Verification items for the finished model (mm, model axes). Face numbers are marked on the shaded views. A direction names the side the tool comes from. Coordinates: 2 decimals unless noted, no trailing zeros. Loops run counter-clockwise (first coordinate to the right, second up) from the corner with the lowest first, then second, coordinate; pieces in that order, holes last. Notation, with made-up numbers: (-36, 15.5) - (-15, 15.5) arc R24 cw to (-15, 43.5) - close; hole circle Ø6 at (5, 29). An arc over 180 degrees is marked (long way). Answer as CSV lines item,"result". Start each with the question number.
1. Cross-section at C-C (y = 4.75). Enter the section's corners in (x, z).
2. Gauge pin test, flat end, axial feed: P1, Ø9, axis at x = 4, y = 5.5, coming from the +Z side. Record the tip position at first contact, or that the pin passes through.
3. Cross-section at B-B (z = 7.5). Enter the section's corners in (x, y).
4. Cross-section at A-A (y = -2.5). Enter the section's corners in (x, z), plus the area to 3 significant figures.
5. Material ranges on line 1 (X direction, y = 0.75, z = 4.5); line 2 (Z direction, x = -3.5, y = 6.75); line 3 (Y direction, x = 16.85, z = 7), recorded low to high. Write a range as [from, to].
6. Release check for a two-part mould opening along X. For the marked faces 1, 2 and 3 record: pulls with the +X half, pulls with the -X half, needs draft (parallel to the pull), parting line crosses it, or undercut.
7. Cross-section at D-D (x = 10.5). Enter the section's corners in (y, z), plus the area to 4 significant figures.
8. Set-up check for the marked faces 4 and 5: record each of +Z, -Z, +X, -X, +Y, -Y from which the full face is reachable in a straight line by a thin tool's end or side.
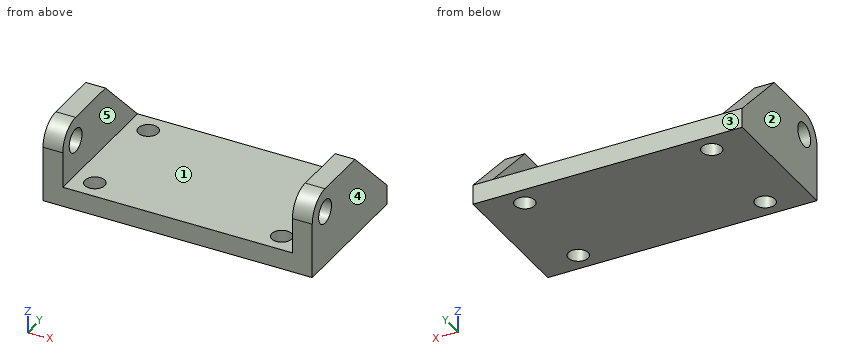
```python
from build123d import *

# Parameters (mm, degrees)
SKETCH1_W           = 34
SKETCH1_H           = 17.5
SKETCH1_R           = 1.25
BOSS_EXTRUDE1_DEPTH = 2.5
SKETCH2_W           = 2.5
SKETCH2_H           = 17.5
BOSS_EXTRUDE2_DEPTH = 7.5
CHAMFER1_SIZE       = 7.5
FILLET1_R           = 3
SKETCH3_R           = 1.5
CUT_EXTRUDE1_DEPTH  = 35


with BuildPart() as part:
    # Sketch1 → Boss-Extrude1 (new body)
    with BuildSketch(Plane.XY):
        with Locations((0.621428571, 4.137142857)):
            Rectangle(SKETCH1_W, SKETCH1_H)
        with Locations((-11.178571429, -2.112857143)):
            Circle(SKETCH1_R, mode=Mode.SUBTRACT)
        with Locations((12.421428571, -2.112857143)):
            Circle(SKETCH1_R, mode=Mode.SUBTRACT)
        with Locations((12.421428571, 10.387142857)):
            Circle(SKETCH1_R, mode=Mode.SUBTRACT)
        with Locations((-11.178571429, 10.387142857)):
            Circle(SKETCH1_R, mode=Mode.SUBTRACT)
    extrude(amount=BOSS_EXTRUDE1_DEPTH)

    # Sketch2 → Boss-Extrude2 (add)
    with BuildSketch(Plane.XY.offset(2.5)):
        with Locations((-15.128571429, 4.137142857)):
            Rectangle(SKETCH2_W, SKETCH2_H)
        with Locations((16.371428571, 4.137142857)):
            Rectangle(SKETCH2_W, SKETCH2_H)
    extrude(amount=BOSS_EXTRUDE2_DEPTH)

    # Chamfer1
    chamfer1_edges = [part.edges().sort_by_distance(p)[0] for p in [
        (16.371428571, 12.887142857, 10),
        (-15.128571429, 12.887142857, 10),
    ]]
    chamfer(chamfer1_edges, length=CHAMFER1_SIZE)

    # Fillet1
    fillet1_edges = [part.edges().sort_by_distance(p)[0] for p in [
        (-15.128571429, -4.612857143, 10),
        (16.371428571, -4.612857143, 10),
    ]]
    fillet(fillet1_edges, radius=FILLET1_R)

    # Sketch3 → Cut-Extrude1 (cut, through all)
    with BuildSketch(Plane(origin=(17.621428571, 0, 0), x_dir=(0, 0, -1), z_dir=(1, 0, 0))):
        with Locations((-7, -1.612857143)):
            Circle(SKETCH3_R)
    extrude(amount=-CUT_EXTRUDE1_DEPTH, mode=Mode.SUBTRACT)


solid = part.part
```
Values follow:
1,outline,"(-16.38, 0) - (17.62, 0) - (17.62, 10) - (15.12, 10) - (15.12, 2.5) - (-13.88, 2.5) - (-13.88, 10) - (-16.38, 10) - close"
2,P1,"stops at z = 2.5"
3,outline,"(-16.38, -4.57) - (-13.88, -4.57) - (-13.88, -3.03) - (-16.38, -3.03) - close; (-16.38, -0.2) - (-13.88, -0.2) - (-13.88, 7.89) - (-16.38, 7.89) - close; (15.12, -4.57) - (17.62, -4.57) - (17.62, -3.03) - (15.12, -3.03) - close; (15.12, -0.2) - (17.62, -0.2) - (17.62, 7.89) - (15.12, 7.89) - close"
4,outline,"(-16.38, 0) - (-12.37, 0) - (-12.37, 2.5) - (-13.88, 2.5) - (-13.88, 5.79) - (-16.38, 5.79) - close; (-16.38, 8.21) - (-13.88, 8.21) - (-13.88, 9.87) - (-16.38, 9.87) - close; (-9.99, 0) - (11.23, 0) - (11.23, 2.5) - (-9.99, 2.5) - close; (13.61, 0) - (17.62, 0) - (17.62, 5.79) - (15.12, 5.79) - (15.12, 2.5) - (13.61, 2.5) - close; (15.12, 8.21) - (17.62, 8.21) - (17.62, 9.87) - (15.12, 9.87) - close"
4,area,"97.8 mm²"
5,line 1,"x = [-16.38, -13.88], [15.12, 17.62]"
5,line 2,"z = [0, 2.5]"
5,line 3,"y = [-4.61, -3.11], [-0.11, 8.39]"
6,face 1,"undercut"
6,face 2,"pulls with the -X half"
6,face 3,"needs draft"
7,outline,"(-4.61, 0) - (12.89, 0) - (12.89, 2.5) - (-4.61, 2.5) - close"
7,area,"43.75 mm²"
8,face 4,"+Z, -Z, +X, +Y, -Y"
8,face 5,"+Z, +Y, -Y"
